from build123d import *

# Parameters (mm, degrees)
CYLINDER008_R               = 1.35
CYLINDER008_DEPTH           = 10
CYLINDER008_PLACEMENT_ANGLE = 91
CYLINDER007_R               = 1.35
CYLINDER007_DEPTH           = 10
CYLINDER007_PITCH_ANGLE     = 90
CYLINDER006_R               = 5
CYLINDER006_DEPTH           = 20
CYLINDER006_PITCH_ANGLE     = 90
BOX001_W                    = 10
BOX001_H                    = 6
BOX001_DEPTH                = 22
CYLINDER005_R               = 10
CYLINDER005_DEPTH           = 110
CUT007_PITCH_ANGLE          = 90
CUT007_PLACEMENT_ANGLE      = -90


with BuildPart() as cylinder008:
    # Cylinder008 → Cylinder008 (new body)
    with BuildSketch(Plane.XY):
        Circle(CYLINDER008_R)
    extrude(amount=CYLINDER008_DEPTH)


with BuildPart() as cylinder008_1:
    # Cylinder008 placement: moved
    add(cylinder008.part.moved(Location((0, 0, 85))).rotate(Axis((0, 0, 85), (0, 1, 0)), CYLINDER008_PLACEMENT_ANGLE))


with BuildPart() as cylinder007:
    # Cylinder007 → Cylinder007 (new body)
    with BuildSketch(Plane.XY):
        Circle(CYLINDER007_R)
    extrude(amount=CYLINDER007_DEPTH)


with BuildPart() as cylinder007_1:
    # Cylinder007 pitch: moved
    add(cylinder007.part.rotate(Axis((0, 0, 0), (0, 1, 0)), CYLINDER007_PITCH_ANGLE))


with BuildPart() as cylinder007_2:
    # Cylinder007 placement: moved
    add(cylinder007_1.part.moved(Location((0, 0, 69))))


with BuildPart() as cylinder006:
    # Cylinder006 → Cylinder006 (new body)
    with BuildSketch(Plane.XY):
        Circle(CYLINDER006_R)
    extrude(amount=CYLINDER006_DEPTH)


with BuildPart() as cylinder006_1:
    # Cylinder006 pitch: moved
    add(cylinder006.part.rotate(Axis((0, 0, 0), (0, 1, 0)), CYLINDER006_PITCH_ANGLE))


with BuildPart() as cylinder006_2:
    # Cylinder006 placement: moved
    add(cylinder006_1.part.moved(Location((-10, 0, 77))))


with BuildPart() as cube001:
    # Box001 → Box001 (new body)
    with BuildSketch(Plane(origin=(9.54, -3, 66), x_dir=(1, 0, 0), z_dir=(0, 0, 1))):
        with Locations((5, 3)):
            Rectangle(BOX001_W, BOX001_H)
    extrude(amount=BOX001_DEPTH)


with BuildPart() as lever002:
    # Cylinder005 → Cylinder005 (new body)
    with BuildSketch(Plane.XY.offset(22)):
        Circle(CYLINDER005_R)
    extrude(amount=CYLINDER005_DEPTH)

    # Cut006: cut Cube001
    add(cube001.part, mode=Mode.SUBTRACT)

    # Cut004: cut Cylinder006
    add(cylinder006_2.part, mode=Mode.SUBTRACT)

    # Cut005: cut Cylinder007
    add(cylinder007_2.part, mode=Mode.SUBTRACT)

    # Cut007: cut Cylinder008
    add(cylinder008_1.part, mode=Mode.SUBTRACT)


with BuildPart() as lever002_1:
    # Cut007 pitch: moved
    add(lever002.part.rotate(Axis((0, 0, 0), (0, 1, 0)), CUT007_PITCH_ANGLE))


with BuildPart() as lever002_2:
    # Cut007 placement: moved
    add(lever002_1.part.moved(Location((0, 77, 0))).rotate(Axis((0, 77, 0), (0, 0, 1)), CUT007_PLACEMENT_ANGLE))


solid = lever002_2.part
Design review of the part built by this model. Coordinates are the model's own, in mm. A direction names the side the tool comes from. Round coordinates to 2 decimals unless told otherwise and drop trailing zeros. Write each loop counter-clockwise with the first axis right and the second up, starting at its lowest first coordinate (ties: lowest second). Pieces come first, ordered by that corner, then holes. Notation, with made-up numbers: (20, 0) -> (59, 0) arc R27 ccw to (59, 29) -> close; hole circle Ø4 at (14, 28.25). An arc over 180 degrees is marked (long way). One line per item, written item: value. Start each with the question number.
Q1. Add section B-B (y = 8). Give the boundary of the cut face in (x, z), then the cut area to 3 significant figures.
Q2. The part is to be moulded in two halves that separate along X. For faces 4 (the face through (0, -55, 0)), 5 (the face through (4.957, -0.651, 0.367)), 6 (the face through (6.76, 0.77, 7.37)), say which applies: pulls with the +X half, pulls with the -X half, needs draft (parallel to the pull), parting line crosses it, or undercut.
Q3. Add section D-D (z = -1.5). State how many separate pieces and enclosed holes the cut face has, then the cut area to 3 significant figures.
Q4. Insertion check: P1, Ø1, axis at x = 3.5, y = 15, coming from the -Z side; P2, Ø3, axis at y = -32.5, z = -3, coming from the +X side; P3, Ø3, axis at x = -4, y = 0.5, coming from the +Z side. Each pin has a flat end and moves straight along its axis. Give the tip position at first contact, or say it passes through.
Q5. Add section C-C (z = 4.5). Give the boundary of the cut face in (x, y).
Q6. To check wall thickness, follow probe 1 along Y at (x, z) = (4, 8.25); probe 2 along Z at (x, y) = (-3.5, 4.5); probe 3 along X at (y, z) = (8, -6). State the ranges of each line that lie inside material, in increasing order.
Q7. Tool access review of faces 1 (the face through (0.41, -6.63, -4.69)), 2 (the face through (-1.4, 6.8, -9.54)), 3 (the face through (0, 8, 0)): name each direction out of +Z, -Z, +X, -X, +Y, -Y from which nothing blocks a thin tool from reaching the whole face with its end or side.
Q8. Add section A-A (x = 0). Give the boundary of the cut face in (y, z), then the cut area to 3 significant figures.
Response:
1. outline: (-3, -9.54) -> (-1.35, -9.54) -> (-1.35, 0) -> (1.35, 0) -> (1.35, -9.54) -> (3, -9.54) arc R10 ccw (long way) to start
1. area: 287 mm^2
2. face 4: needs draft
2. face 5: undercut
2. face 6: parting line crosses it
3. separate pieces: 1
3. enclosed holes: 3
3. area: 2,090 mm^2
4. P1: stops at z = -9.54
4. P2: stops at x = 9.89
4. P3: stops at z = 8.86
5. outline: (-8.93, -55) -> (8.93, -55) -> (8.93, 55) -> (-8.93, 55) -> close; hole circle Ø10 at (0, 0)
6. probe 1: y = -55 to -3, 3 to 55
6. probe 2: z = -9.37 to 9.37
6. probe 3: x = -8 to -1.35, 1.35 to 8
7. face 1: none
7. face 2: -Z, +X, -X
7. face 3: -Z
8. outline: (-55, -10) -> (-11, -10) -> (-11, -9.54) -> (-9.18, -9.54) -> (-9.35, -0.02) -> (-6.65, 0.02) -> (-6.48, -9.54) -> (-5, -9.54) -> (-5, 10) -> (-55, 10) -> close; (5, -9.54) -> (6.65, -9.54) -> (6.65, 0) -> (9.35, 0) -> (9.35, -9.54) -> (11, -9.54) -> (11, -10) -> (55, -10) -> (55, 10) -> (5, 10) -> close
8. area: 1,940 mm^2
